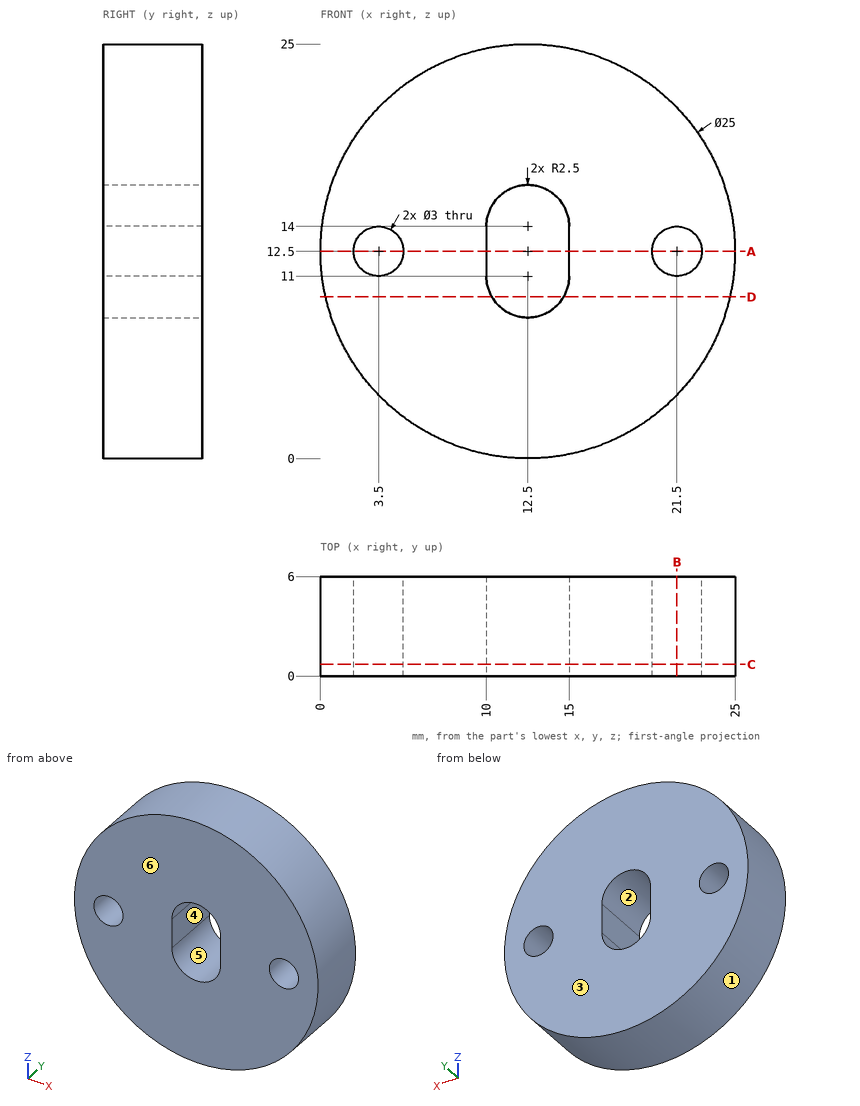
Study the drawing (mm; zero at the part's minimum x, y, z) and answer. A direction names the side the tool comes from. Give positions to 0.01 mm unless a question says otherwise; leave off trailing zeros. Loops run counter-clockwise (first coordinate to the right, second up) from the corner with the lowest first, then second, coordinate; pieces in that order, holes last. Notation, with made-up numbers: (21, 4) -> (67, 4) arc R27 cw to (67, 42) -> close; hole circle Ø3 at (21, 54.25). An arc over 180 degrees is marked (long way). Write item = value, one per line. Start each with the question number.
(1) Find section D-D on z = 9.75. Give the vertices of the cut face in (x, y), and give its area (3 significant figures).
(2) Which of the six approach directions +Z, -Z, +X, -X, +Y, -Y give full straight-line access (tool end or side, diameter ignored) to the marked faces 5 and 6?
(3) Find section B-B on x = 21.5. Give the vertices of the cut face in (y, z).
(4) Find the intervals of material crossed by probe 1 along X at (y, z) = (4, 12.5); probe 2 along X at (y, z) = (1.5, 2.5); probe 3 along Z at (x, y) = (2.5, 4.1), in increasing order. Write a range as from..to.
(5) Find section A-A on z = 12.5. Give the vertices of the cut face in (x, y).
(6) The mould has two halves that part along Z. Classify the marked faces 1, 2, 3 and 4: +Z half, -Z half, draft (parallel to the pull), parting line (faces both ways), or undercut.
(7) Given pin 1 Ø1.5 at (y, z) = (1.5, 3.5) entering from +X; pin 2 Ø1 at (x, y) = (11, 4.5) entering from -Z; pin 3 Ø3 at (y, z) = (1.5, 16.5) entering from +X, each flat-ended and moving along its own axis, determine where each tip first touches the part or whether it passes through.
(8) Find section C-C on y = 0.7. Give the vertices of the cut face in (x, z).
From the geometry:
q1.outline = (0.31, 0) -> (10.33, 0) -> (10.33, 6) -> (0.31, 6) -> close; (14.67, 0) -> (24.69, 0) -> (24.69, 6) -> (14.67, 6) -> close
q1.area = 120 mm^2
q2.face_5 = +Y, -Y
q2.face_6 = +Z, -Z, +X, -X, -Y
q3.outline = (0, 3.83) -> (6, 3.83) -> (6, 11) -> (0, 11) -> close; (0, 14) -> (6, 14) -> (6, 21.17) -> (0, 21.17) -> close
q4.probe_1 = 0..2, 5..10, 15..20, 23..25
q4.probe_2 = 5..20
q4.probe_3 = 5..11.38, 13.62..20
q5.outline = (0, 0) -> (2, 0) -> (2, 6) -> (0, 6) -> close; (5, 0) -> (10, 0) -> (10, 6) -> (5, 6) -> close; (15, 0) -> (20, 0) -> (20, 6) -> (15, 6) -> close; (23, 0) -> (25, 0) -> (25, 6) -> (23, 6) -> close
q6.face_1 = parting line
q6.face_2 = undercut
q6.face_3 = draft
q6.face_4 = undercut
q7.pin_1 = 21.89
q7.pin_2 = 0.04
q7.pin_3 = 24.75
q8.outline = circle Ø25 at (12.5, 12.5); hole circle Ø3 at (3.5, 12.5); hole (10, 11) arc R2.5 ccw to (15, 11) -> (15, 14) arc R2.5 ccw to (10, 14) -> close; hole circle Ø3 at (21.5, 12.5)
